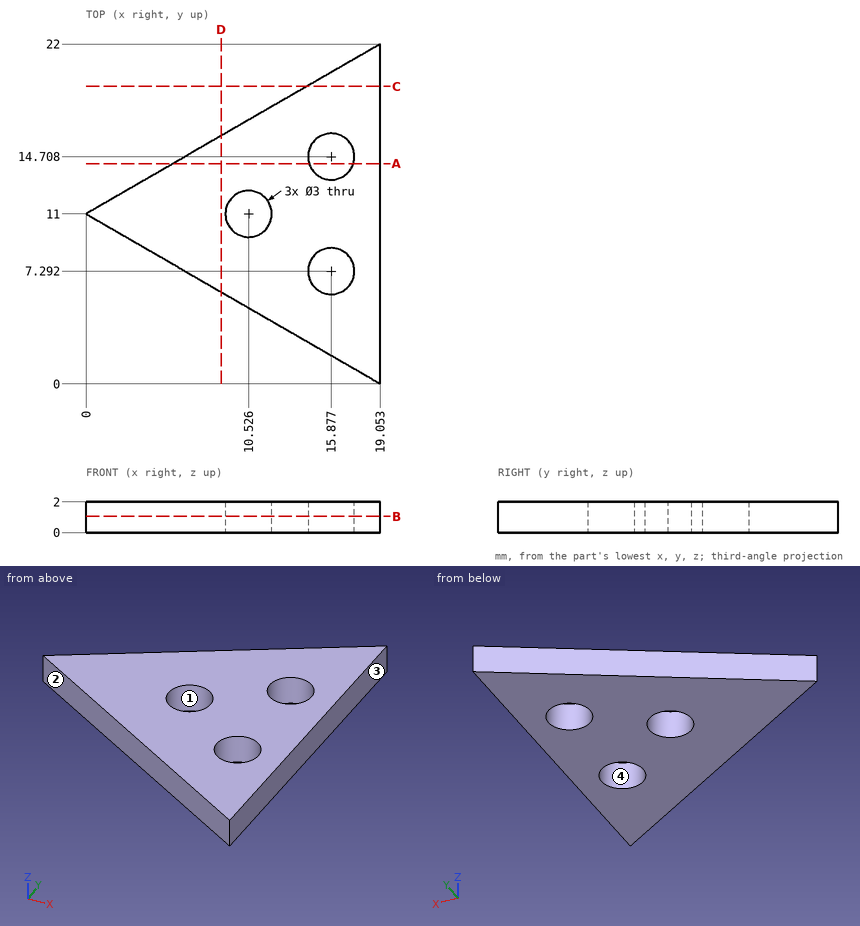
Here's the drawing with two shaded views (mm, measured from the low corner). I have some questions. Coordinates: 2 decimals unless noted, no trailing zeros. Write each loop counter-clockwise with the first axis right and the second up, starting at its lowest first coordinate (ties: lowest second). Pieces come first, ordered by that corner, then holes. Notation, with made-up numbers: M 76.25,17.25 L 87.25,17.25 A15 ccw 87.25,34.25 Z; hole C -5.75,-16.5 d4. An arc over 180 degrees is marked long. Answer as CSV lines item,"result".
Item 1: Imagine slicing it at A-A on y = 14.25. List the corners of the cut face in (x, z) for me (1 decimal).
Geometry results:
outline,"M 5.6,0 L 14.4,0 L 14.4,2 L 5.6,2 Z; M 17.3,0 L 19.1,0 L 19.1,2 L 17.3,2 Z"
Item 2: Imagine slicing it at D-D on x = 8.75. List the corners of the cut face in (y, z) for me.
Geometry results:
outline,"M 5.95,0 L 16.05,0 L 16.05,2 L 5.95,2 Z"
Item 3: We'd pull the mould along Y, two halves only. Please class the marked faces 1, 2, 3 and 4: +Y half, -Y half, draft (parallel to the pull), parting line (faces both ways), or undercut.
Geometry results:
face 1,"undercut"
face 2,"-Y half"
face 3,"draft"
face 4,"undercut"
Item 4: Imagine slicing it at C-C on y = 19.25. List the corners of the cut face in (x, z) for me.
Geometry results:
outline,"M 14.29,0 L 19.05,0 L 19.05,2 L 14.29,2 Z"
Item 5: Imagine slicing it at B-B on z = 1.05. List the corners of the cut face in (x, y) for me.
Geometry results:
outline,"M 0,11 L 19.05,0 L 19.05,22 Z; hole C 10.53,11 d3; hole C 15.88,7.29 d3; hole C 15.88,14.71 d3"
Item 6: Please list where these lines run through material, in increasing order: line 1 along Y through (x, z) = (17.25, 1.7) (1 decimal); line 2 along Y through (x, z) = (16.5, 1.1) (1 decimal); line 3 along Y through (x, z) = (10.75, 0.25) (1 decimal).
Geometry results:
line 1,"y = 1 to 6.7, 7.9 to 14.1, 15.3 to 21"
line 2,"y = 1.5 to 5.9, 8.7 to 13.3, 16.1 to 20.5"
line 3,"y = 4.8 to 9.5, 12.5 to 17.2"
Item 7: I'm going to push a flat-ended pin straight in: P1, Ø4, axis at x = 10.53, y = 11, coming from the -Z side. Where does the tip first touch, or does it pass through?
Geometry results:
P1,"stops at z = 0"
